Answer from the drawing. Dimensions are ordinates in mm from the lowest x, y and z of the part. Round coordinates to 2 decimals unless told otherwise and drop trailing zeros. Loops run counter-clockwise (first coordinate to the right, second up) from the corner with the lowest first, then second, coordinate; pieces in that order, holes last. Notation, with made-up numbers: (22.5, 26.5) - (76.5, 26.5) arc R29 ccw to (76.5, 61.5) - close; hole circle Ø1 at (44.5, 83.25). An arc over 180 degrees is marked (long way). Answer as CSV lines item,"result".
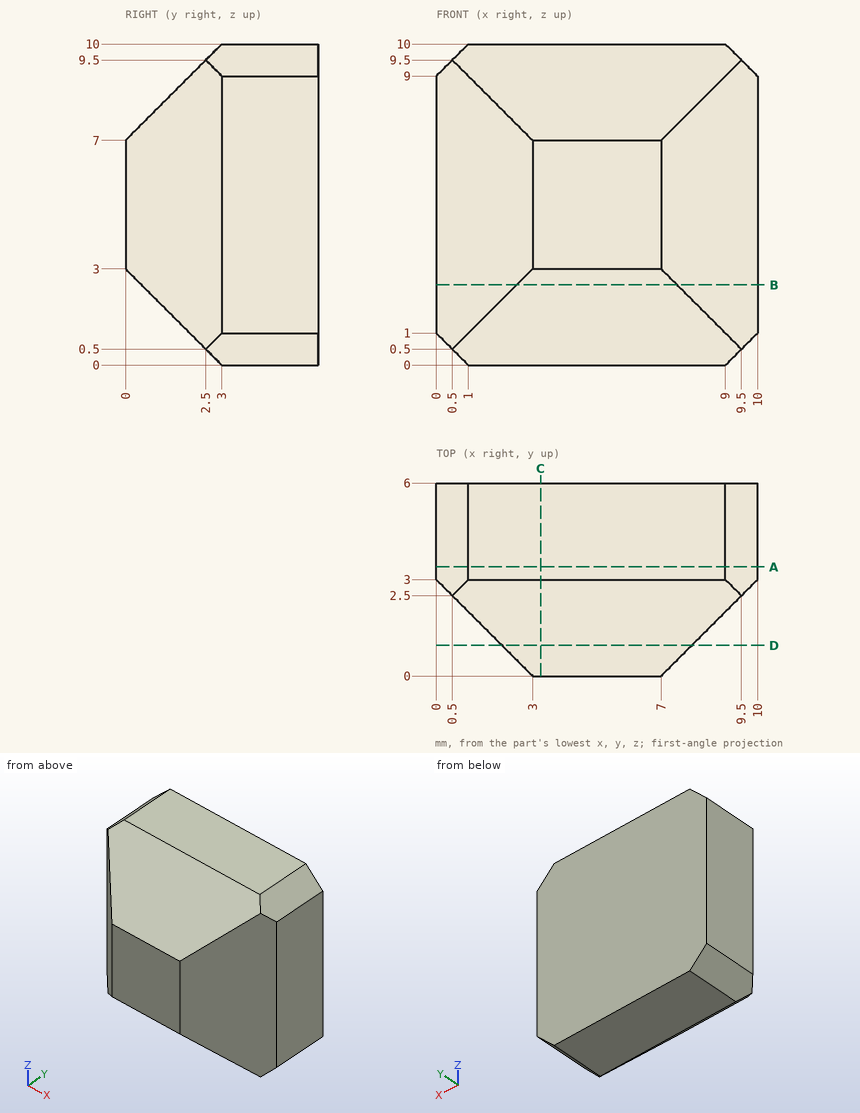
1) A cutting plane is placed at D-D, the plane y = 0.95. Determine the outline of the cut face in (x, z), plus the area to 3 significant figures.
Entries:
outline,"(2.05, 2.05) - (7.95, 2.05) - (7.95, 7.95) - (2.05, 7.95) - close"
area,"34.8 mm^2"
2) A cutting plane is placed at A-A, the plane y = 3.4. Determine the outline of the cut face in (x, z), plus the area to 3 significant figures.
Entries:
outline,"(0, 1) - (1, 0) - (9, 0) - (10, 1) - (10, 9) - (9, 10) - (1, 10) - (0, 9) - close"
area,"98.0 mm^2"
3) A cutting plane is placed at C-C, the plane x = 3.25. Determine the outline of the cut face in (y, z).
Entries:
outline,"(0, 3) - (3, 0) - (6, 0) - (6, 10) - (3, 10) - (0, 7) - close"
4) Find the intervals of material crossed by line 1 (X direction, y = 3.8, z = 0.5); line 2 (Z direction, x = 4.5, y = 2); line 3 (Y direction, x = 0.5, z = 5.25), in increasing order.
Entries:
line 1,"x = 0.5 to 9.5"
line 2,"z = 1 to 9"
line 3,"y = 2.5 to 6"
5) A cutting plane is placed at B-B, the plane z = 2.5. Determine the outline of the cut face in (x, y).
Entries:
outline,"(0, 3) - (2.5, 0.5) - (7.5, 0.5) - (10, 3) - (10, 6) - (0, 6) - close"
6) Each of these flat-tipped pins is pushed along its axis until it touches: P1, Ø1.5, axis at y = 1.5, z = 3.5, coming from the -X side; P2, Ø2, axis at y = 1.5, z = 8.5, coming from the -X side. Where does it stop, or does it pass through?
Entries:
P1,"stops at x = 0.75"
P2,"stops at x = 0.5"
